from build123d import *

# Parameters (mm, degrees)
SKETCH1_W                 = 40
SKETCH1_H                 = 8
BOSS_EXTRUDE1_DEPTH       = 3
F_8_CLEARANCE_HOLE1_D     = 4.4958
F_8_CLEARANCE_HOLE1_DEPTH = 17
F_8_CLEARANCE_HOLE1_TIP   = 1.350674586
SKETCH5_W                 = 2
SKETCH5_H                 = 8
BOSS_EXTRUDE2_DEPTH       = 5
BOSS_EXTRUDE2_DEPTH_BACK  = 8
SKETCH6_R                 = 2
CUT_EXTRUDE1_DEPTH        = 2


with BuildPart() as part:
    # Sketch1 → Boss-Extrude1 (new body)
    with BuildSketch(Plane(origin=(0, 0, 0), x_dir=(1, 0, 0), z_dir=(0, 1, 0))):
        with Locations((12.773632998, 0.313559322)):
            Rectangle(SKETCH1_W, SKETCH1_H)
    extrude(amount=BOSS_EXTRUDE1_DEPTH)

    # #8 Clearance Hole1
    with Locations(Plane(origin=(0.773632998, 3, -0.313559322), x_dir=(0, 0, 1), z_dir=(0, 1, 0))):
        with Locations((0, 0), (0, 24)):
            Hole(F_8_CLEARANCE_HOLE1_D / 2, depth=F_8_CLEARANCE_HOLE1_DEPTH)
            with Locations((0, 0, -(F_8_CLEARANCE_HOLE1_DEPTH + F_8_CLEARANCE_HOLE1_TIP / 2))):  # 118° drill point
                Cone(0, F_8_CLEARANCE_HOLE1_D / 2, F_8_CLEARANCE_HOLE1_TIP, mode=Mode.SUBTRACT)

    # Sketch5 → Boss-Extrude2 (add, two sides)
    with BuildSketch(Plane(origin=(0, 3, 0), x_dir=(1, 0, 0), z_dir=(0, 1, 0))) as boss_extrude2_sk:
        with Locations((13.773632998, 0.313559322)):
            Rectangle(SKETCH5_W, SKETCH5_H)
    extrude(amount=BOSS_EXTRUDE2_DEPTH)
    extrude(boss_extrude2_sk.sketch, amount=-BOSS_EXTRUDE2_DEPTH_BACK)

    # Sketch6 → Cut-Extrude1 (cut)
    with BuildSketch(Plane.ZY.offset(-12.773632998)):
        with Locations((-0.313559322, 5.5)):
            Circle(SKETCH6_R)
        with Locations((-0.313559322, -2.5)):
            Circle(SKETCH6_R)
    extrude(amount=-CUT_EXTRUDE1_DEPTH, mode=Mode.SUBTRACT)


solid = part.part
Could you check a few things on this model? Use its own coordinates, in mm. A direction names the side the tool comes from. Round coordinates to 2 decimals unless told otherwise and drop trailing zeros. Order: outer loops, then holes, each group sorted by start corner. A loop starts at its lowest first (then second) coordinate and runs counter-clockwise, first axis right, second up.
(1) Imagine slicing it at D-D (x = 10). Write out the boundary of the cut face in (y, z).
Response values:
outline: (0, -4.31) - (3, -4.31) - (3, 3.69) - (0, 3.69) - close
(2) Which directions (+Z, -Z, +X, -X, +Y, -Y) give clear straight access to the entire face, cutting with the end or side of a thin tool? Please do faces 1 (the flat face through (3, 3, -2)), 2 (the flat face through (3, 0, -2)), 3 (the flat face through (22, 3, 0)).
Response values:
face 1: +Z, -Z, -X, +Y
face 2: +Z, -Z, -X, -Y
face 3: +Z, -Z, +X, +Y
(3) Imagine slicing it at C-C (x = 25.5). Write out the boundary of the cut face in (y, z).
Response values:
outline: (0, -4.31) - (3, -4.31) - (3, -2.44) - (0, -2.44) - close; (0, 1.81) - (3, 1.81) - (3, 3.69) - (0, 3.69) - close
(4) Imagine slicing it at A-A (y = 5.5). Write out the boundary of the cut face in (x, z), plus the area to 3 significant figures.
Response values:
outline: (12.77, -4.31) - (14.77, -4.31) - (14.77, -2.31) - (12.77, -2.31) - close; (12.77, 1.69) - (14.77, 1.69) - (14.77, 3.69) - (12.77, 3.69) - close
area: 8.00 mm2
(5) If we mould it in two halves opening along Z, with no side actions, what happens to faces 4 (the flat face through (22, 0, 0)), 5 (the flat face through (13, 2, 3.686)), 6 (the cylindrical face through (27, 1, 0)), 7 (the flat face through (13, 1, -4.314))? For each: released by +Z, released by -Z, zero draft, split by the parting line, or undercut.
Response values:
face 4: zero draft
face 5: released by +Z
face 6: undercut
face 7: released by -Z
(6) Please list where these lines run through material, in increasing order: line 1 along X through (y, z) = (2.25, 1.5); line 2 along Y through (x, z) = (17.5, 1.5); line 3 along X through (y, z) = (-0.25, 0.25).
Response values:
line 1: x = -7.23 to -0.55, 2.1 to 23.45, 26.1 to 32.77
line 2: y = 0 to 3
line 3: x = 12.77 to 14.77
(7) I'm going to push flat-ended pins straight in: pin 1 (4 mm diameter, centred on y = 6, z = 1, fed in from -X); pin 2 (4 mm diameter, centred on x = 23.5, z = 1.5, fed in from +Y). Where does each tip first touch, or does it pass through?
Response values:
pin 1: stops at x = 12.77
pin 2: stops at y = 3
(8) Imagine slicing it at B-B (z = -1.5). Write out the boundary of the cut face in (x, y), plus the area to 3 significant figures.
Response values:
outline: (-7.23, 0) - (-1.14, 0) - (-1.14, 3) - (-7.23, 3) - close; (2.68, 0) - (12.77, 0) - (12.77, -0.89) - (14.77, -0.89) - (14.77, 0) - (22.86, 0) - (22.86, 3) - (14.77, 3) - (14.77, 3.89) - (12.77, 3.89) - (12.77, 3) - (2.68, 3) - close; (12.77, -5) - (14.77, -5) - (14.77, -4.11) - (12.77, -4.11) - close; (12.77, 7.11) - (14.77, 7.11) - (14.77, 8) - (12.77, 8) - close; (26.68, 0) - (32.77, 0) - (32.77, 3) - (26.68, 3) - close
area: 104 mm2
